Geometry: final body of the model. Coordinates: model frame, mm. Give positions to 0.01 mm unless a question says otherwise; leave off trailing zeros. Use one line per item in the form item = value. Start each with the question number.
Item 1: Section query A-A on z = 228.5. Give the number of separate pieces and of enclosed holes in the cut face, then the cut area to 3 significant figures.
Item 2: Material intervals for line 1 along Y through (x, z) = (0, 122); line 2 along Y through (x, z) = (-0.5, 100); line 3 along Y through (x, z) = (-8.5, 187) (3 decimals), sorted ascending. Write a range as from..to.
Item 3: Contact query for flat-ended pins moving along their axis: P1, Ø6.5, axis at x = 0, y = -20, coming from the +Z side; P2, Ø1, axis at y = -18.5, z = 151, coming from the -X side; P3, Ø4, axis at y = -20.5, z = 63.5, coming from the +X side. Output: stop coordinate, or through.
from build123d import *

# Parameters (mm, degrees)
SKETCH1_R           = 2.1
BOSS_EXTRUDE1_DEPTH = 380


with BuildPart() as part:
    # Sketch1 → Boss-Extrude1 (new body)
    with BuildSketch(Plane.XY):
        with BuildLine():
            Line((4.58, -30), (9.5, -30))
            ThreePointArc((9.5, -30), (9.853553391, -29.853553391), (10, -29.5))
            Line((10, -29.5), (10, -24.58))
            Line((10, -24.58), (8.545, -23.125))
            Line((8.545, -23.125), (8.2, -23.125))
            Line((8.2, -23.125), (8.2, -25.5))
            Line((8.2, -25.5), (6.560660172, -25.5))
            Line((6.560660172, -25.5), (3.9, -22.839339828))
            Line((3.9, -22.839339828), (3.9, -20.21))
            Line((3.9, -20.21), (3.69, -20))
            Line((3.69, -20), (3.9, -19.79))
            Line((3.9, -19.79), (3.9, -17.160660172))
            Line((3.9, -17.160660172), (6.560660172, -14.5))
            Line((6.560660172, -14.5), (8.2, -14.5))
            Line((8.2, -14.5), (8.2, -16.875))
            Line((8.2, -16.875), (8.545, -16.875))
            Line((8.545, -16.875), (10, -15.42))
            Line((10, -15.42), (10, -4.58))
            Line((10, -4.58), (8.545, -3.125))
            Line((8.545, -3.125), (8.2, -3.125))
            Line((8.2, -3.125), (8.2, -5.5))
            Line((8.2, -5.5), (6.560660172, -5.5))
            Line((6.560660172, -5.5), (3.9, -2.839339828))
            Line((3.9, -2.839339828), (3.9, -0.21))
            Line((3.9, -0.21), (3.69, 0))
            Line((3.69, 0), (3.9, 0.21))
            Line((3.9, 0.21), (3.9, 2.839339828))
            Line((3.9, 2.839339828), (6.560660172, 5.5))
            Line((6.560660172, 5.5), (8.2, 5.5))
            Line((8.2, 5.5), (8.2, 3.125))
            Line((8.2, 3.125), (8.545, 3.125))
            Line((8.545, 3.125), (10, 4.58))
            Line((10, 4.58), (10, 15.42))
            Line((10, 15.42), (8.545, 16.875))
            Line((8.545, 16.875), (8.2, 16.875))
            Line((8.2, 16.875), (8.2, 14.5))
            Line((8.2, 14.5), (6.560660172, 14.5))
            Line((6.560660172, 14.5), (3.9, 17.160660172))
            Line((3.9, 17.160660172), (3.9, 19.79))
            Line((3.9, 19.79), (3.69, 20))
            Line((3.69, 20), (3.9, 20.21))
            Line((3.9, 20.21), (3.9, 22.839339828))
            Line((3.9, 22.839339828), (6.560660172, 25.5))
            Line((6.560660172, 25.5), (8.2, 25.5))
            Line((8.2, 25.5), (8.2, 23.125))
            Line((8.2, 23.125), (8.545, 23.125))
            Line((8.545, 23.125), (10, 24.58))
            Line((10, 24.58), (10, 29.5))
            ThreePointArc((10, 29.5), (9.853553391, 29.853553391), (9.5, 30))
            Line((9.5, 30), (4.58, 30))
            Line((4.58, 30), (3.125, 28.545))
            Line((3.125, 28.545), (3.125, 28.2))
            Line((3.125, 28.2), (5.5, 28.2))
            Line((5.5, 28.2), (5.5, 26.560660172))
            Line((5.5, 26.560660172), (2.839339828, 23.9))
            Line((2.839339828, 23.9), (0.21, 23.9))
            Line((0.21, 23.9), (0, 23.69))
            Line((0, 23.69), (-0.21, 23.9))
            Line((-0.21, 23.9), (-2.839339828, 23.9))
            Line((-2.839339828, 23.9), (-5.5, 26.560660172))
            Line((-5.5, 26.560660172), (-5.5, 28.2))
            Line((-5.5, 28.2), (-3.125, 28.2))
            Line((-3.125, 28.2), (-3.125, 28.545))
            Line((-3.125, 28.545), (-4.58, 30))
            Line((-4.58, 30), (-9.5, 30))
            ThreePointArc((-9.5, 30), (-9.853553391, 29.853553391), (-10, 29.5))
            Line((-10, 29.5), (-10, 24.58))
            Line((-10, 24.58), (-8.545, 23.125))
            Line((-8.545, 23.125), (-8.2, 23.125))
            Line((-8.2, 23.125), (-8.2, 25.5))
            Line((-8.2, 25.5), (-6.560660172, 25.5))
            Line((-6.560660172, 25.5), (-3.9, 22.839339828))
            Line((-3.9, 22.839339828), (-3.9, 20.21))
            Line((-3.9, 20.21), (-3.69, 20))
            Line((-3.69, 20), (-3.9, 19.79))
            Line((-3.9, 19.79), (-3.9, 17.160660172))
            Line((-3.9, 17.160660172), (-6.560660172, 14.5))
            Line((-6.560660172, 14.5), (-8.2, 14.5))
            Line((-8.2, 14.5), (-8.2, 16.875))
            Line((-8.2, 16.875), (-8.545, 16.875))
            Line((-8.545, 16.875), (-10, 15.42))
            Line((-10, 15.42), (-10, 4.58))
            Line((-10, 4.58), (-8.545, 3.125))
            Line((-8.545, 3.125), (-8.2, 3.125))
            Line((-8.2, 3.125), (-8.2, 5.5))
            Line((-8.2, 5.5), (-6.560660172, 5.5))
            Line((-6.560660172, 5.5), (-3.9, 2.839339828))
            Line((-3.9, 2.839339828), (-3.9, 0.21))
            Line((-3.9, 0.21), (-3.69, 0))
            Line((-3.69, 0), (-3.9, -0.21))
            Line((-3.9, -0.21), (-3.9, -2.839339828))
            Line((-3.9, -2.839339828), (-6.560660172, -5.5))
            Line((-6.560660172, -5.5), (-8.2, -5.5))
            Line((-8.2, -5.5), (-8.2, -3.125))
            Line((-8.2, -3.125), (-8.545, -3.125))
            Line((-8.545, -3.125), (-10, -4.58))
            Line((-10, -4.58), (-10, -15.42))
            Line((-10, -15.42), (-8.545, -16.875))
            Line((-8.545, -16.875), (-8.2, -16.875))
            Line((-8.2, -16.875), (-8.2, -14.5))
            Line((-8.2, -14.5), (-6.560660172, -14.5))
            Line((-6.560660172, -14.5), (-3.9, -17.160660172))
            Line((-3.9, -17.160660172), (-3.9, -19.79))
            Line((-3.9, -19.79), (-3.69, -20))
            Line((-3.69, -20), (-3.9, -20.21))
            Line((-3.9, -20.21), (-3.9, -22.839339828))
            Line((-3.9, -22.839339828), (-6.560660172, -25.5))
            Line((-6.560660172, -25.5), (-8.2, -25.5))
            Line((-8.2, -25.5), (-8.2, -23.125))
            Line((-8.2, -23.125), (-8.545, -23.125))
            Line((-8.545, -23.125), (-10, -24.58))
            Line((-10, -24.58), (-10, -29.5))
            ThreePointArc((-10, -29.5), (-9.853553391, -29.853553391), (-9.5, -30))
            Line((-9.5, -30), (-4.58, -30))
            Line((-4.58, -30), (-3.125, -28.545))
            Line((-3.125, -28.545), (-3.125, -28.2))
            Line((-3.125, -28.2), (-5.5, -28.2))
            Line((-5.5, -28.2), (-5.5, -26.560660172))
            Line((-5.5, -26.560660172), (-2.839339828, -23.9))
            Line((-2.839339828, -23.9), (-0.21, -23.9))
            Line((-0.21, -23.9), (0, -23.69))
            Line((0, -23.69), (0.21, -23.9))
            Line((0.21, -23.9), (2.839339828, -23.9))
            Line((2.839339828, -23.9), (5.5, -26.560660172))
            Line((5.5, -26.560660172), (5.5, -28.2))
            Line((5.5, -28.2), (3.125, -28.2))
            Line((3.125, -28.2), (3.125, -28.545))
            Line((3.125, -28.545), (4.58, -30))
        make_face()
        with Locations((0, -20)):
            Circle(SKETCH1_R, mode=Mode.SUBTRACT)
        Polygon((-6.239339828, -12.7), (-8.2, -12.7), (-8.2, -7.3), (-6.239339828, -7.3), (-2.839339828, -3.9), (2.839339828, -3.9), (6.239339828, -7.3), (8.2, -7.3), (8.2, -12.7), (6.239339828, -12.7), (2.839339828, -16.1), (-2.839339828, -16.1), align=None, mode=Mode.SUBTRACT)
        Polygon((-6.239339828, 7.3), (-8.2, 7.3), (-8.2, 12.7), (-6.239339828, 12.7), (-2.839339828, 16.1), (2.839339828, 16.1), (6.239339828, 12.7), (8.2, 12.7), (8.2, 7.3), (6.239339828, 7.3), (2.839339828, 3.9), (-2.839339828, 3.9), align=None, mode=Mode.SUBTRACT)
        with Locations((0, 20)):
            Circle(SKETCH1_R, mode=Mode.SUBTRACT)
        Circle(SKETCH1_R, mode=Mode.SUBTRACT)
    extrude(amount=BOSS_EXTRUDE1_DEPTH)


solid = part.part
Answer sheet:
q1.separate_pieces = 1
q1.enclosed_holes = 5
q1.area = 429 mm2
q2.line_1 = -23.69..-22.1, -17.9..-16.1, -3.9..-2.1, 2.1..3.9, 16.1..17.9, 22.1..23.69
q2.line_2 = -23.9..-22.04, -17.96..-16.1, -3.9..-2.04, 2.04..3.9, 16.1..17.96, 22.04..23.9
q2.line_3 = -30..-23.125, -16.875..-3.125, 3.125..16.875, 23.125..30
q3.P1 = 380
q3.P2 = -3.9
q3.P3 = 3.9
